Autodesk Inventor part; units mm, degrees
ref_plane "YZ Plane" through (0, 0, 0) normal (1, 0, 0) x (0, 1, 0)
ref_plane "XZ Plane" through (0, 0, 0) normal (0, 1, 0) x (-1, 0, 0)
ref_plane "XY Plane" through (0, 0, 0) normal (0, 0, 1) x (1, 0, 0)
sketch "Эскиз1" plane through (0, 0, 0) normal (0, 1, 0) x (-1, 0, 0)
  circle A0 centre (0, 8) radius 1.85
  circle A1 centre (0, -8) radius 1.85
  line L0 (0, -8) -> (0, -13)
  line L1 (0, -13) -> (5, -13)
  line L2 (5, -13) -> (5, 43)
  line L3 (5, 43) -> (0, 43)
  line L4 (0, 43) -> (0, -13)
  line L5 (0, -13) -> (-5, -13)
  line L6 (-5, -13) -> (-5, 43)
  line L7 (-5, 43) -> (0, 43)
  line L8 (5, -13) -> (10, -13)
  line L9 (10, -13) -> (10, 43)
  line L10 (10, 43) -> (5, 43)
  line L11 (5, 43) -> (5, -13)
  line L12 (-5, -13) -> (-10, -13)
  line L13 (-10, -13) -> (-10, 43)
  line L14 (-10, 43) -> (-5, 43)
  line L15 (-5, 43) -> (-5, -13)
  point P0 (0, 0)
  dimension "d0" = 5
  dimension "d2" = 56
extrude "Выдавливание1" add sketch "Эскиз1" along normal blind 3.2 contours A0 L4 L3 L2 L1 L0 A1 | A0 L4 A1 L0 L5 L6 L7 | L10 L9 L8 L2 | L6 L12 L13 L14
sketch "Эскиз2" plane through (0, 0, 0) normal (0, -1, 0) x (1, 0, 0)
  line L0 (-10, 43) -> (10, 43)
  line L1 (-10, 43) -> (10, 43)
  line L2 (10, 43) -> (10, 39.8)
  line L3 (10, 39.8) -> (-10, 39.8)
  line L4 (-10, 39.8) -> (-10, 43)
  point P0 (0, 0)
  dimension "d9" = 20
  dimension "d10" = 3.2
extrude "Выдавливание2" add sketch "Эскиз2" against normal blind 10
sketch "Эскиз3" plane through (0, 10, 0) normal (0, 1, 0) x (1, 0, 0)
  line L0 (10, -39.8) -> (-10, -39.8)
  line L1 (-10, -39.8) -> (-10, -43)
  line L2 (-10, -43) -> (10, -43)
  line L3 (10, -43) -> (10, -39.8)
  point P0 (0, 0)
extrude "Выдавливание3" add sketch "Эскиз3" along normal blind 1.2
sketch "Эскиз4" plane through (-10, 0, 43) normal (0, 0, 1) x (1, 0, 0)
  point P0 (10, 0)
sketch "Эскиз5" plane through (-10, 0, 43) normal (0, 0, 1) x (1, 0, 0)
  ellipse E0 centre (6.0228, 6.7252) end of major axis (6.0228, 4.4752) minor radius 2.2495 (8.0223, 5.6944) -> (4.0232, 5.6944) ccw
  ellipse E1 centre (15.9206, 6.7252) end of major axis (15.9206, 8.9752) minor radius 2.2495 (17.9202, 5.6944) -> (13.921, 5.6944) ccw
  circle A0 centre (6.0228, 6.7252) radius 2.25
  circle A1 centre (15.9206, 6.7252) radius 2.25
  point P0 (10, 0)
  point P1 (15.9206, 8.9752)
  point P2 (15.9696, 8.975)
  point P3 (6.0719, 8.975)
  point P4 (6.0228, 8.9752)
extrude "Выдавливание4" cut sketch "Эскиз5" against normal through all
sketch "Эскиз6" plane through (10, 0, 43) normal (1, 0, 0) x (0, 0, -1)
  line L0 (0, 0) -> (56, 0)
  line L1 (56, 0) -> (56, 3.2)
  line L2 (3.2, 3.2) -> (56, 3.2)
  line L3 (3.2, 3.2) -> (3.2, 11.2)
  line L4 (0, 11.2) -> (3.2, 11.2)
  line L5 (0, 0) -> (0, 11.2)
  line L6 (3.2, 11.2) -> (16, 3.2)
  point P0 (43, 0)
extrude "Выдавливание5" add sketch "Эскиз6" along normal blind 3.2
sketch "Эскиз7" plane through (-10, 0, -13) normal (-1, 0, 0) x (0, 0, 1)
  line L0 (52.8, 3.2) -> (52.8, 11.2)
  line L1 (40, 3.2) -> (52.8, 11.2)
  line L2 (52.8, 3.2) -> (40, 3.2)
  line L3 (0, 3.2) -> (52.8, 3.2)
  line L4 (0, 0) -> (0, 3.2)
  line L5 (0, 0) -> (56, 0)
  line L6 (56, 0) -> (56, 11.2)
  line L7 (52.8, 11.2) -> (56, 11.2)
  line L8 (52.8, 3.2) -> (52.8, 11.2)
  point P0 (13, 0)
extrude "Выдавливание6" add sketch "Эскиз7" along normal blind 3.2
ref_plane "РабПлоскость1" through (0, 0, -13) normal (1, 0, 0) x (0, 0, -1)
sketch "Эскиз8" plane through (0, 0, -13) normal (1, 0, 0) x (0, 0, -1)
  line L0 (-40, 3.2) -> (-52.8, 3.2)
  line L1 (-52.8, 11.2) -> (-40, 3.2)
  line L2 (-52.8, 3.2) -> (-52.8, 11.2)
  point P0 (-13, 0)
extrude "Выдавливание7" add sketch "Эскиз8" along normal blind 1
sketch "Эскиз9" plane through (0, 0, -13) normal (-1, 0, 0) x (0, 0, 1)
  line L0 (52.8, 11.2) -> (52.8, 3.2)
  line L1 (40, 3.2) -> (52.8, 11.2)
  line L2 (52.8, 3.2) -> (40, 3.2)
  point P0 (13, 0)
extrude "Выдавливание8" add sketch "Эскиз9" along normal blind 1
fillet "Сопряжение1" radius 2 4 edges at (10, 3.2, 33.4) (-10, 3.2, 33.4) (1, 3.2, 33.4) (-1, 3.2, 33.4)
sketch "Эскиз10" plane through (0, 0, 0) normal (0, -1, 0) x (1, 0, 0)
  line L0 (-3.0752, 19.5502) -> (-3.0021, 23.0495)
  arc A0 (3.9956, 22.9433) -> (3.5069, 23.4136) centre (3.4965, 22.9137) ccw
  line L1 (9.496, 22.8284) -> (3.9956, 22.9433)
  line L2 (9.9129, 42.784) -> (9.496, 22.8284)
  line L3 (-8.0832, 43.16) -> (9.9129, 42.784)
  line L4 (-8.0832, 43.16) -> (-8.5001, 23.2044)
  line L5 (-2.9997, 23.0894) -> (-8.5001, 23.2044)
  arc A1 (-2.4918, 23.5389) -> (-2.9997, 23.0894) centre (-2.5022, 23.039) ccw
  line L6 (-2.4918, 23.5389) -> (3.5069, 23.4136)
  line L7 (-3.0752, 19.5502) -> (-3.0021, 23.0495)
  line L8 (-8.5009, 23.1644) -> (-3.0021, 23.0495)
  line L9 (-8.584, 19.1852) -> (-8.5009, 23.1644)
  line L10 (-2.7253, 19.0628) -> (-8.584, 19.1852)
  arc A2 (-3.0752, 19.5502) -> (-2.7253, 19.0628) centre (-2.5753, 19.5398) ccw
  arc A3 (3.5533, 18.9317) -> (3.9233, 19.404) centre (3.4234, 19.4145) ccw
  line L11 (9.412, 18.8093) -> (3.5533, 18.9317)
  line L12 (9.412, 18.8093) -> (9.4952, 22.7884)
  line L13 (3.9964, 22.9033) -> (9.4952, 22.7884)
  line L14 (3.9964, 22.9033) -> (3.9233, 19.404)
  line L15 (-8.0067, 17.5728) -> (-4.9183, 17.5083)
  line L16 (-4.9183, 17.5083) -> (-4.9475, 16.1086)
  line L17 (-4.9475, 16.1086) -> (5.6502, 15.8872)
  line L18 (5.6502, 15.8872) -> (5.6794, 17.2869)
  line L19 (5.6794, 17.2869) -> (8.7679, 17.2224)
  line L20 (9.4912, 18.8003) -> (8.7679, 17.2224)
  ellipse E0 centre (9.3638, 16.5021) end of major axis (9.412, 18.8093) minor radius 1 (9.4912, 18.8003) -> (9.412, 18.8093) ccw
  line L21 (9.412, 18.8093) -> (3.5533, 18.9317)
  line L22 (3.5533, 18.9317) -> (-2.7253, 19.0628)
  line L23 (-2.7253, 19.0628) -> (-8.584, 19.1852)
  ellipse E1 centre (-8.6322, 16.878) end of major axis (-8.584, 19.1852) minor radius 1 (-8.584, 19.1852) -> (-8.6635, 19.1796) ccw
  line L24 (-8.0067, 17.5728) -> (-8.6635, 19.1796)
  line L25 (3.4376, 23.4704) -> (-15, 23.4704)
  line L26 (-15, 23.4704) -> (-15, 18.9749)
  line L27 (-15, 18.9749) -> (3.4376, 18.9749)
  line L28 (3.4376, 18.9749) -> (3.4376, 23.4704)
  point P0 (0, 0)
extrude "Выдавливание9" cut sketch "Эскиз10" against normal through all contours A2 L10 L9 L8 L0 | L0 L8 L9 E1 L24 L27 L26 L25 L4 L5 A1 L6 L28 L22 A2 | L22 L27 L24 E1 L10 | L6 L25 L28 | L25 A1 L5 L4
fillet "Сопряжение2" radius 2 2 edges at (3.4376, 1.6, 23.4704) (3.4376, 1.6, 18.9749)
fillet "Сопряжение3" radius 2 4 edges at (13.2, 1.6, -13) (-13.2, 1.6, -13) (-13.2, 1.6, 23.4704) (-13.2, 1.6, 18.9749)
fillet "Сопряжение4" radius 2 1 edges at (0, 0, 43)
sketch "Эскиз11" plane through (0, 0, 0) normal (0, -1, 0) x (1, 0, 0)
  line L0 (3.4376, 21.4704) -> (3.4376, 20.9749)
  line L1 (3.4376, 21.2226) -> (-14.4424, 21.2226)
  line L2 (3.4376, 21.2226) -> (-13.5624, 21.2226)
  line L3 (-13.5624, 21.2226) -> (-13.5624, 21.9726)
  line L4 (-13.5624, 21.9726) -> (3.4376, 21.9726)
  line L5 (3.4376, 21.9726) -> (3.4376, 21.2226)
  line L6 (-13.5624, 21.2226) -> (-13.5624, 20.4726)
  line L7 (-13.5624, 20.4726) -> (3.4376, 20.4726)
  line L8 (3.4376, 20.4726) -> (3.4376, 21.2226)
  circle A0 centre (0, -8) radius 1.85
  circle A1 centre (0, 8) radius 1.85
  line L9 (-13.2, 41) -> (13.2, 41)
  line L10 (-13.2, 25.4704) -> (-13.2, 41)
  arc A2 (-13.2, 25.4704) -> (-11.2, 23.4704) centre (-11.2, 25.4704) ccw
  line L11 (-11.2, 23.4704) -> (1.4376, 23.4704)
  arc A3 (3.4376, 21.4704) -> (1.4376, 23.4704) centre (1.4376, 21.4704) ccw
  line L12 (3.4376, 21.4704) -> (3.4376, 20.9749)
  arc A4 (1.4376, 18.9749) -> (3.4376, 20.9749) centre (1.4376, 20.9749) ccw
  line L13 (1.4376, 18.9749) -> (-11.2, 18.9749)
  arc A5 (-11.2, 18.9749) -> (-13.2, 16.9749) centre (-11.2, 16.9749) ccw
  line L14 (-13.2, -11) -> (-13.2, 16.9749)
  arc A6 (-13.2, -11) -> (-11.2, -13) centre (-11.2, -11) ccw
  line L15 (-11.2, -13) -> (11.2, -13)
  arc A7 (11.2, -13) -> (13.2, -11) centre (11.2, -11) ccw
  line L16 (13.2, 41) -> (13.2, -11)
  line L17 (-13.2, 16.9749) -> (-13.2, -11)
  line L18 (-13.2, 25.4704) -> (-13.2, 16.9749)
  point P0 (0, 0)
  point P1 (-13.2, 21.9726)
  point P2 (3.3735, 21.9726)
  point P3 (3.3735, 20.4726)
  point P4 (-13.2, 20.4726)
  dimension "d30" = 17
  dimension "d31" = 0.75
extrude "Выдавливание10" add sketch "Эскиз11" against normal up to surface (3.2 mm away) contours L4 L18 A2 L11 A3 | A4 L13 A5 L18 L7
fillet "Сопряжение5" radius 2 2 edges at (-13.2, 1.6, 20.4726) (-13.2, 1.6, 21.9726)
properties part number "для захвата"
Verification items for the finished model (mm, model axes). A direction names the side the tool comes from. Coordinates: 2 decimals unless noted, no trailing zeros. Loops run counter-clockwise (first coordinate to the right, second up) from the corner with the lowest first, then second, coordinate; pieces in that order, holes last. Notation, with made-up numbers: (45.5, -22.5) - (94.5, -22.5) arc R27 ccw to (94.5, 8.5) - close; hole circle Ø2 at (22.25, 81). An arc over 180 degrees is marked (long way). Answer as a JSON object with one key per item and string values.
(1) Cross-section at B-B, the plane z = 8. Record the boundary of the cut face in (x, y), then the cut area to 3 significant figures.
Response:
{"outline": "(-13.2, 0) - (-1.85, 0) - (-1.85, 3.2) - (-13.2, 3.2) - close; (1.85, 0) - (13.2, 0) - (13.2, 3.2) - (1.85, 3.2) - close", "area": "72.6 mm²"}
(2) Go/stop test with flat-tipped pins: pin 1 Ø6 at (x, z) = (0, -8) entering from +Y; pin 2 Ø4 at (x, y) = (5, 8.5) entering from -Z; pin 3 Ø0.5 at (y, z) = (2, 21) entering from -X. Record where each tip stops, or that it passes through.
Response:
{"pin 1": "stops at y = 3.2", "pin 2": "stops at z = 39.8", "pin 3": "stops at x = 3.42"}
(3) Cross-section at A-A, the plane x = 0. Record the boundary of the cut face in (y, z), then the cut area to 3 significant figures.
Response:
{"outline": "(0, -13) - (3.2, -13) - (3.2, -9.85) - (0, -9.85) - close; (0, -6.15) - (3.2, -6.15) - (3.2, 6.15) - (0, 6.15) - close; (0, 9.85) - (3.2, 9.85) - (3.2, 20.47) - (0, 20.47) - close; (0, 21.97) - (3.2, 21.97) - (3.2, 27) - (11.2, 39.8) - (11.2, 43) - (2, 43) arc R2 ccw to (0, 41) - close", "area": "227 mm²"}
(4) Cross-section at D-D, the plane z = 32. Record the boundary of the cut face in (x, y) (3 decimals), then the cut area to 3 significant figures.
Response:
{"outline": "(-13.2, 0) - (13.2, 0) - (13.2, 6.325) - (10, 6.325) - (10, 5.2) arc R2 cw to (8, 3.2) - (3, 3.2) arc R2 cw to (1, 5.2) - (1, 6.325) - (-1, 6.325) - (-1, 5.2) arc R2 cw to (-3, 3.2) - (-8, 3.2) arc R2 cw to (-10, 5.2) - (-10, 6.325) - (-13.2, 6.325) - close", "area": "114 mm²"}
(5) Cross-section at C-C, the plane y = 10. Record the boundary of the cut face in (x, z), then the cut area to 3 significant figures.
Response:
{"outline": "(-13.2, 37.88) - (-10, 37.88) - (-10, 39.8) - (-1, 39.8) - (-1, 37.88) - (1, 37.88) - (1, 39.8) - (10, 39.8) - (10, 37.88) - (13.2, 37.88) - (13.2, 43) - (-13.2, 43) - close", "area": "101 mm²"}
(6) Scan lines: line 1 along Z through (x, y) = (0, 2.05); line 2 along X through (y, z) = (7, 37); line 3 along X through (y, z) = (1.55, 8). Record each from-to range of solid material in increasing order.
Response:
{"line 1": "z = -13 to -9.85, -6.15 to 6.15, 9.85 to 20.47, 21.97 to 43", "line 2": "x = -13.2 to -10, -1 to 1, 10 to 13.2", "line 3": "x = -13.2 to -1.85, 1.85 to 13.2"}
(7) Mould release check, pull along X, two halves, no side actions. Record for faces 1 (the flat face through (1, 7, 37)), 2 (the cylindrical face through (-12.599, 1.622, 22.543)), 3 (the cylindrical face through (0.18, 0.6, 42.43)): pulls with the +X half, pulls with the -X half, needs draft (parallel to the pull), parting line crosses it, or undercut.
Response:
{"face 1": "undercut", "face 2": "pulls with the -X half", "face 3": "needs draft"}
(8) Access from +Z, -Z, +X, -X, +Y, -Y to the whole of each face (thin tool, end or side, straight path). Record for faces 4 (the cylindrical face through (0.401, 1.578, -6.194)), 5 (the cylindrical face through (-9.43, 3.8, 33.49)), 6 (the cylindrical face through (12.63, 1.62, -12.4)), 7 (the cylindrical face through (5.886, 4.475, 41.422)), 8 (the flat face through (-4, 2, 20.473)).
Response:
{"face 4": "+Y, -Y", "face 5": "-Z, +Y", "face 6": "-Z, +X, +Y, -Y", "face 7": "+Z, -Z", "face 8": "-X, +Y, -Y"}
